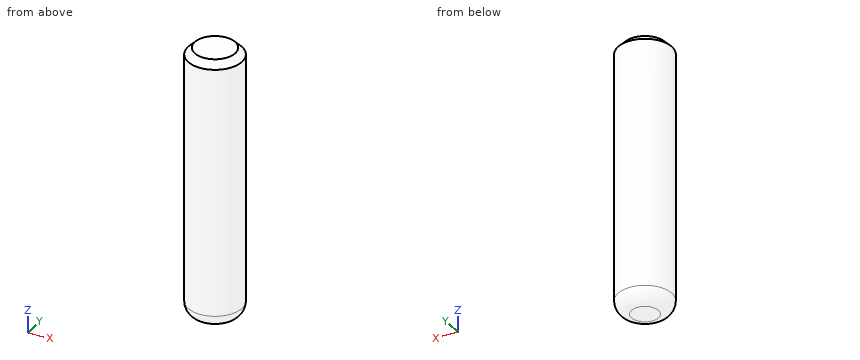
Autodesk Inventor part; units mm, degrees
ref_plane "YZ Plane" through (0, 0, 0) normal (1, 0, 0) x (0, 1, 0)
ref_plane "XZ Plane" through (0, 0, 0) normal (0, 1, 0) x (-1, 0, 0)
ref_plane "XY Plane" through (0, 0, 0) normal (0, 0, 1) x (1, 0, 0)
sketch "Sketch1" plane through (0, 0, 0) normal (0, 0, 1) x (1, 0, 0)
  circle A0 centre (0, 0) radius 2
  dimension "d0" = 4
extrude "Extrusion1" add sketch "Sketch1" along normal mid plane 20
fillet "Fillet1" radius 1 1 edges at (-2, 0, -10)
chamfer "Chamfer1" distance 0.5 angle 45 1 edges at (-2, 0, 10)
properties part number "DOWEL,M4X20" material "Steel"
The model under review builds one solid part; all positions refer to its coordinate system, in mm. Coordinates: 2 decimals unless noted, no trailing zeros. Loops run counter-clockwise (first coordinate to the right, second up) from the corner with the lowest first, then second, coordinate; pieces in that order, holes last. Notation, with made-up numbers: (64.25, 62.25) -> (81.25, 62.25) arc R18 ccw to (81.25, 87.25) -> close; hole circle Ø7 at (32.25, 31). An arc over 180 degrees is marked (long way). Answer as CSV lines item,"result".
Item 1: For L1, parallel to X at y = -1.6, z = -7; L2, parallel to X at y = 0.25, z = 8.5; L3, parallel to Y at x = -0.15, z = 7, list the stretches that pass through material, from the lowest coordinate up.
Results below:
L1,"x = -1.2 to 1.2"
L2,"x = -1.98 to 1.98"
L3,"y = -1.99 to 1.99"
Item 2: Insertion check: pin 1 (1 mm diameter, centred on x = -1.5, z = -3, fed in from +Y); pin 2 (2 mm diameter, centred on y = 0.5, z = -4, fed in from -X); pin 3 (1 mm diameter, centred on x = -1, z = -0.5, fed in from -Y). Each pin has a flat end and moves straight along its axis. Give the tip position at first contact, or say it passes through.
Results below:
pin 1,"stops at y = 1.73"
pin 2,"stops at x = -2"
pin 3,"stops at y = -1.94"
Item 3: Take a section at A-A, the plane z = 5.25. State the section outline as (x, y) points, and give its area (3 significant figures).
Results below:
outline,"circle Ø4 at (0, 0)"
area,"12.6 mm2"
